The listing builds one solid part. Answer for the finished solid, in the listing's coordinates (mm). Round coordinates to 2 decimals unless told otherwise and drop trailing zeros. Write each loop counter-clockwise with the first axis right and the second up, starting at its lowest first coordinate (ties: lowest second). Pieces come first, ordered by that corner, then holes. Notation, with made-up numbers: M 68,5.5 L 89,5.5 A32 cw 89,43.5 Z; hole C 56,68 d7. An arc over 180 degrees is marked long. One line per item, written item: value. Start each with the question number.
(1) Section B-B (z = -105.5) is taken. Determine the outline of the cut face in (x, y), plus the area to 3 significant figures.
(2) Section A-A (x = -73.5) is taken. Determine the outline of the cut face in (y, z), plus the area to 3 significant figures.
(3) Section C-C (y = 1.25) is taken. State how many separate pieces and enclosed holes the cut face has, plus the area to 3 significant figures.
(4) Consider probe 1 along Z at (x, y) = (-20.5, 1.6); probe 2 along Z at (x, y) = (-28, 2.5); probe 3 along Z at (x, y) = (-50.5, 0.45). Determine where each line is inside the solid, lowest interval first.
(5) Given P1, Ø2.5, axis at x = -111.2, z = -105.5, coming from the +Y side; P2, Ø2.5, axis at y = 1.5, z = -116.5, coming from the -X side; P3, Ø1.2, axis at y = 3, z = -59.5, coming from the -X side; P4, Ø2.5, axis at y = 2, z = -90.5, coming from the +X side, each flat-ended and moving along its own axis, determine where each tip first touches the part or whether it passes through.
(6) Section D-D (z = -22.5) is taken. Determine the outline of the cut face in (x, y).
Autodesk Inventor part; units mm, degrees
ref_plane "YZ Plane" through (0, 0, 0) normal (1, 0, 0) x (0, 1, 0)
ref_plane "XZ Plane" through (0, 0, 0) normal (0, 1, 0) x (-1, 0, 0)
ref_plane "XY Plane" through (0, 0, 0) normal (0, 0, 1) x (1, 0, 0)
sketch "Sketch1" plane through (0, 0, 0) normal (0, 1, 0) x (-1, 0, 0)
  line L0 (0, 0) -> (116.2, 0)
  line L1 (116.2, 0) -> (116.2, -56.7)
  line L2 (116.2, -56.7) -> (42, -56.7)
  line L3 (2, -18) -> (94.2, -18)
  line L4 (96.2, -20) -> (96.2, -36.75)
  line L5 (94.2, -38.75) -> (2, -38.75)
  arc A0 (96.2, -20) -> (94.2, -18) centre (94.2, -20) ccw
  arc A1 (94.2, -38.75) -> (96.2, -36.75) centre (94.2, -36.75) ccw
  line L6 (0, -56.75) -> (0, -40.75)
  line L7 (0, -16) -> (0, 0)
  arc A2 (0, -16) -> (2, -18) centre (2, -16) ccw
  arc A3 (2, -38.75) -> (0, -40.75) centre (2, -40.75) ccw
  line L8 (151.2965, -59.25) -> (-22.324, -59.25) construction
  line L9 (0, -118.5) -> (116.2, -118.5)
  line L10 (116.2, -118.5) -> (116.2, -61.8)
  line L11 (116.2, -61.8) -> (42, -61.8)
  line L12 (2, -100.5) -> (94.2, -100.5)
  line L13 (96.2, -98.5) -> (96.2, -81.75)
  line L14 (94.2, -79.75) -> (2, -79.75)
  arc A4 (94.2, -100.5) -> (96.2, -98.5) centre (94.2, -98.5) ccw
  arc A5 (96.2, -81.75) -> (94.2, -79.75) centre (94.2, -81.75) ccw
  line L15 (0, -61.75) -> (0, -77.75)
  line L16 (0, -102.5) -> (0, -118.5)
  arc A6 (2, -100.5) -> (0, -102.5) centre (2, -102.5) ccw
  arc A7 (0, -77.75) -> (2, -79.75) centre (2, -77.75) ccw
  line L17 (40, -58.7) -> (40, -59.8)
  line L18 (0, -61.75) -> (0, -56.75)
  arc A8 (40, -59.8) -> (42, -61.8) centre (42, -59.8) ccw
  arc A9 (42, -56.7) -> (40, -58.7) centre (42, -58.7) ccw
  point P0 (96.2, -38.75)
  point P1 (96.2, -18)
  point P2 (0, -38.75)
  point P3 (0, -28.375)
  point P4 (96.2, -79.75)
  point P5 (96.2, -100.5)
  point P6 (0, -79.75)
  point P7 (0, -90.125)
  dimension "d3" = 20.75
  dimension "d4" = 2
  dimension "d11" = 2
  dimension "d26" = 2
  dimension "d27" = 59.25
  dimension "d28" = 59.25
  dimension "d29" = 116.2
  dimension "d30" = 20
  dimension "d31" = 5.1
  dimension "d32" = 2.55
  dimension "d33" = 40
  dimension "d34" = 18
extrude "Extrusion1" add sketch "Sketch1" along normal blind 5
sketch "Sketch3" plane through (0, 5, 0) normal (0, 1, 0) x (1, 0, 0)
  line L0 (-141.9344, 59.25) -> (33.9299, 59.25) construction
  line L1 (0, 40.75) -> (0, 77.75) construction
  line L2 (-141.9344, 66.75) -> (21.3081, 66.75) construction
  line L3 (-111.2, -34.402) -> (-111.2, 125.7551) construction
  line L4 (-130.4345, 113.5) -> (5.6009, 113.5) construction
  line L5 (-141.9344, 5) -> (8.4057, 5) construction
  line L6 (-116.2, 0) -> (0, 0) construction
  line L7 (0, 118.5) -> (-116.2, 118.5) construction
  line L8 (-150.0685, 51.75) -> (12.052, 51.75) construction
  line L9 (-16, -62.5764) -> (-16, 180.6044) construction
  line L10 (0, 102.5) -> (0, 118.5) construction
  line L11 (-73.5, -39.5766) -> (-73.5, 137.6901) construction
  line L12 (-73.5, -38.2066) -> (-73.5, 155.6811) construction
  line L13 (-116.2, 56.7) -> (-116.2, 0)
  point P0 (0, 59.25)
  point P1 (-111.2, 13)
  point P2 (-111.2, 43.75)
  point P3 (-111.2, 74.75)
  point P4 (-111.2, 105.5)
  point P5 (-16, 5)
  point P6 (-16, 113.5)
  point P7 (-16, 66.75)
  point P8 (-73.5, 66.75)
  point P9 (-28, 51.75)
  point P10 (-73.5, 5)
  dimension "d35" = 5
  dimension "d36" = 5
  dimension "d37" = 7.5
  dimension "d38" = 13
  dimension "d39" = 15.5
  dimension "d40" = 15.5
  dimension "d41" = 13
  dimension "d42" = 7.5
  dimension "d43" = 16
  dimension "d44" = 12
  dimension "d45" = 73.5
  dimension "d53" = 73.5
  dimension "d54" = 5
hole "Hole1" at (-111.2, 5, -13) at (-111.2, 5, -43.75) at (-111.2, 5, -74.75) at (-111.2, 5, -105.5) at (-16, 5, -5) at (-16, 5, -113.5) at (-16, 5, -66.75) at (-73.5, 5, -66.75) at (-28, 5, -51.75) at (-73.5, 5, -5) direction (0, -1, 0) diameter 3.8 end through all
sketch "Sketch4" plane through (0, 5, 0) normal (0, 1, 0) x (1, 0, 0)
  line L0 (-116.2, 52.75) -> (-49, 52.75)
  line L1 (-48, 53.75) -> (-48, 64.75)
  line L2 (-49, 65.75) -> (-116.2, 65.75)
  line L3 (-116.2, 65.75) -> (-116.2, 52.75)
  line L4 (-144.8708, 59.25) -> (29.3106, 59.25) construction
  line L5 (-40, 59.8) -> (-40, 58.7) construction
  line L6 (0, 40.75) -> (0, 77.75)
  line L7 (0, 102.5) -> (0, 118.5)
  arc A0 (-48, 64.75) -> (-49, 65.75) centre (-49, 64.75) ccw
  arc A1 (-49, 52.75) -> (-48, 53.75) centre (-49, 53.75) ccw
  line L8 (-116.2, 59.25) -> (-48, 59.25)
  line L9 (0, 118.5) -> (-116.2, 118.5)
  line L10 (-116.2, 118.5) -> (-48, 118.5)
  line L11 (-48, 118.5) -> (-48, 115.5)
  line L12 (-49, 114.5) -> (-116.2, 114.5)
  line L13 (-116.2, 114.5) -> (-116.2, 118.5)
  arc A2 (-49, 114.5) -> (-48, 115.5) centre (-49, 115.5) ccw
  circle A3 centre (-28, 51.75) radius 1.9
  circle A4 centre (-16, 66.75) radius 1.9
  circle A5 centre (-16, 5) radius 1.9
  circle A6 centre (-111.2, 74.75) radius 1.9
  circle A7 centre (-111.2, 13) radius 1.9
  circle A8 centre (-111.2, 43.75) radius 1.9
  circle A9 centre (-111.2, 105.5) radius 1.9
  circle A10 centre (-16, 113.5) radius 1.9
  circle A11 centre (-73.5, 66.75) radius 1.9
  circle A12 centre (-73.5, 5) radius 1.9
  line L14 (-2, 18) -> (-94.2, 18)
  arc A13 (-96.2, 20) -> (-94.2, 18) centre (-94.2, 20) ccw
  line L15 (-96.2, 20) -> (-96.2, 36.75)
  arc A14 (-94.2, 38.75) -> (-96.2, 36.75) centre (-94.2, 36.75) ccw
  line L16 (-94.2, 38.75) -> (-2, 38.75)
  arc A15 (-2, 38.75) -> (0, 40.75) centre (-2, 40.75) ccw
  line L17 (0, 40.75) -> (0, 77.75)
  arc A16 (0, 77.75) -> (-2, 79.75) centre (-2, 77.75) ccw
  line L18 (-2, 79.75) -> (-94.2, 79.75)
  arc A17 (-96.2, 81.75) -> (-94.2, 79.75) centre (-94.2, 81.75) ccw
  line L19 (-96.2, 81.75) -> (-96.2, 98.5)
  arc A18 (-94.2, 100.5) -> (-96.2, 98.5) centre (-94.2, 98.5) ccw
  line L20 (-94.2, 100.5) -> (-2, 100.5)
  arc A19 (-2, 100.5) -> (0, 102.5) centre (-2, 102.5) ccw
  line L21 (0, 102.5) -> (0, 118.5)
  line L22 (0, 118.5) -> (-116.2, 118.5)
  line L23 (-116.2, 118.5) -> (-116.2, 61.8)
  line L24 (-116.2, 61.8) -> (-42, 61.8)
  arc A20 (-40, 59.8) -> (-42, 61.8) centre (-42, 59.8) ccw
  line L25 (-40, 59.8) -> (-40, 58.7)
  arc A21 (-42, 56.7) -> (-40, 58.7) centre (-42, 58.7) ccw
  line L26 (-42, 56.7) -> (-116.2, 56.7)
  line L27 (-116.2, 56.7) -> (-116.2, 0)
  line L28 (-116.2, 0) -> (0, 0)
  line L29 (0, 0) -> (0, 16)
  arc A22 (0, 16) -> (-2, 18) centre (-2, 16) ccw
  point P0 (-40, 59.25)
  dimension "d55" = 48
  dimension "d57" = 6.5
  dimension "d58" = 13
  dimension "d64" = 4
extrude "Extrusion2" cut sketch "Sketch4" against normal blind 5 contours L3 L26 L1 A1 L0 | L3 L8 L1 L26 | L13 L9 L11 A2 L12
sketch "Sketch5" plane through (0, 5, 0) normal (0, 1, 0) x (1, 0, 0)
  line L0 (-6.5, 90.3299) -> (-6.5, 26.5621) construction
  line L1 (0, 40.75) -> (0, 77.75)
  line L2 (-18, 59.25) -> (18, 59.25) construction
  point P0 (0, 0)
  point P1 (0, 59.25)
  point P2 (0, 59.25)
  point P3 (-6.5, 72.75)
  point P4 (-6.5, 45.75)
  dimension "d66" = 6.5
  dimension "d67" = 13.5
  dimension "d68" = 13.5
hole "Hole2" at (-6.5, 5, -72.75) at (-6.5, 5, -45.75) direction (0, -1, 0) diameter 3.8 end through all
properties part number "Battery Top Plate"
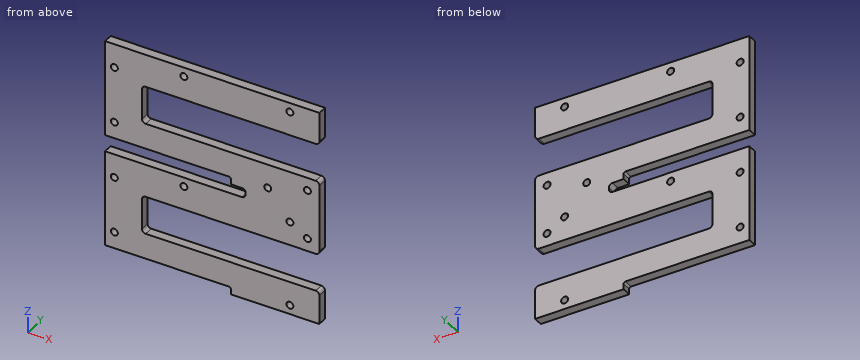
Recorded:
1. outline: M -116.2,0 L -113.1,0 L -113.1,5 L -116.2,5 Z; M -109.3,0 L 0,0 L 0,5 L -109.3,5 Z
1. area: 562 mm2
2. outline: M 0,-114.5 L 5,-114.5 L 5,-100.5 L 0,-100.5 Z; M 0,-79.75 L 5,-79.75 L 5,-68.65 L 0,-68.65 Z; M 0,-64.85 L 5,-64.85 L 5,-61.8 L 0,-61.8 Z; M 0,-52.75 L 5,-52.75 L 5,-38.75 L 0,-38.75 Z; M 0,-18 L 5,-18 L 5,-6.9 L 0,-6.9 Z; M 0,-3.1 L 5,-3.1 L 5,0 L 0,0 Z
2. area: 282 mm2
3. separate pieces: 1
3. enclosed holes: 12
3. area: 8,710 mm2
4. probe 1: z = -118.5 to -100.5, -79.75 to -38.75, -18 to 0
4. probe 2: z = -118.5 to -100.5, -79.75 to -53.65, -49.85 to -38.75, -18 to 0
4. probe 3: z = -114.5 to -100.5, -79.75 to -61.8, -52.75 to -38.75, -18 to 0
5. P1: passes through
5. P2: stops at x = -48.03
5. P3: stops at x = -40.02
5. P4: stops at x = -96.2
6. outline: M -116.2,0 L -96.2,0 L -96.2,5 L -116.2,5 Z
